The model under review builds one solid part; all positions refer to its coordinate system, in mm. Face numbers are marked on the shaded views. A direction names the side the tool comes from. Round coordinates to 2 decimals unless told otherwise and drop trailing zeros. Order: outer loops, then holes, each group sorted by start corner. A loop starts at its lowest first (then second) coordinate and runs counter-clockwise, first axis right, second up. Notation, with made-up numbers: (-38, 55.5) -> (3, 55.5) arc R16 cw to (3, 63.5) -> close; hole circle Ø10 at (72, -5.75). An arc over 180 degrees is marked (long way). Put each result on its own line as item: value. Start each with the question number.
Autodesk Inventor part; units mm, degrees
ref_plane "YZ Plane" through (0, 0, 0) normal (1, 0, 0) x (0, 1, 0)
ref_plane "XZ Plane" through (0, 0, 0) normal (0, 1, 0) x (-1, 0, 0)
ref_plane "XY Plane" through (0, 0, 0) normal (0, 0, 1) x (1, 0, 0)
sketch "Sketch1" plane through (0, 0, 0) normal (0, 0, 1) x (1, 0, 0)
  line L0 (-15.978, -4.8) -> (15.978, -4.8)
  line L1 (15.978, -4.8) -> (15.978, 4.8)
  line L2 (15.978, 4.8) -> (-15.978, 4.8)
  line L3 (-15.978, 4.8) -> (-15.978, -4.8)
  line L4 (-15.978, -4.8) -> (15.978, 4.8) construction
  line L5 (15.978, -4.8) -> (-15.978, 4.8) construction
  point P0 (0, 0)
  dimension "d0" = 31.956
  dimension "d1" = 9.6
extrude "Extrusion1" add sketch "Sketch1" along normal mid plane 15.928
sketch "Sketch2" plane through (-15.978, 4.8, 7.964) normal (0, 1, 0) x (1, 0, 0)
  circle A0 centre (3.957, 3.957) radius 2.45
  point P0 (15.978, 7.964)
  dimension "d4" = 4.9
extrude "Extrusion2" add sketch "Sketch2" along normal blind 2.1
pattern_linear "Rectangular Pattern1" count 4 spacing 8.014 along (1, 0, 0) of "Extrusion2"
mirror "Mirror1" about plane through (0, 0, 0) normal (0, 0, 1) of "Extrusion2", "Rectangular Pattern1"
sketch "Sketch3" plane through (-12.021, 6.9, 4.007) normal (0, 1, 0) x (1, 0, 0)
  point P0 (12.021, 4.007)
shell "Shell1" thickness 1.557 removed faces 1 at (-5.326, -4.8, 2.6547)
sketch "Sketch4" plane through (-15.978, -4.8, 7.964) normal (0, -1, 0) x (1, 0, 0)
  point P0 (15.978, -7.964)
sketch "Sketch6" plane through (-14.421, 3.243, -6.407) normal (0, -1, 0) x (1, 0, 0)
  circle A0 centre (22.435, 6.407) radius 3.267
  circle A1 centre (22.435, 6.407) radius 2.467
  point P0 (14.421, 6.407)
  point P1 (30.399, -1.557)
  dimension "d13" = 6.534
  dimension "d14" = 0.8
extrude "Extrusion3" add sketch "Sketch6" along normal blind 3
pattern_linear "Rectangular Pattern2" count 3 spacing 8.014 along (-1, 0, 0) of "Extrusion3"
properties part number "Lego Brick"
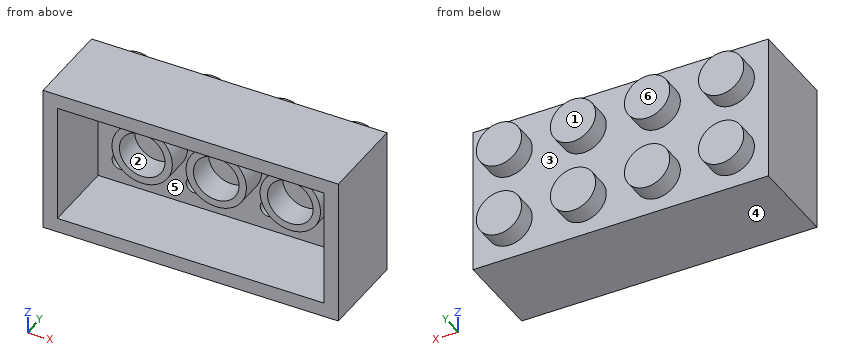
Q1. Draft analysis for pull direction Z (two halves, no side actions). For the marked faces 4, 5 and 6, state which applies: +Z half, -Z half, draft (parallel to the pull), parting line (faces both ways), or undercut.
Q2. For the marked faces 1, 2 and 3, list the 3-axis set-ups (+Z, -Z, +X, -X, +Y, -Y) from which the entire face can be reached by the end or side of a thin tool; tool diameter is ignored.
Q3. Take a section at A-A on y = 1.5. Give the boundary of the cut face in (x, z).
Q4. Wall thickness on probe 1 along Z at (x, y) = (0, 1.9); probe 2 along X at (y, z) = (-1.25, -2.25); probe 3 along Z at (x, y) = (11.5, -3): over which ranges is each line inside the solid? List them lowest first. Write a range as [from, to].
Q5. Take a section at C-C on y = -2.5. Give the boundary of the cut face in (x, z), and give its area (3 significant figures).
Q6. Clearance check with flat-ended pins moving along their axes: pin 1 Ø1.5 at (x, z) = (-8.5, -1) entering from -Y; pin 2 Ø4.5 at (x, z) = (0, 0) entering from +Y; pin 3 Ø1.4 at (x, z) = (4, -4) entering from -Y. State where each tip first meets the part, or that it passes through.
Q7. Take a section at B-B on x = 0. Give the boundary of the cut face in (y, z).
Calculated:
1. face 4: -Z half
1. face 5: undercut
1. face 6: draft
2. face 1: +Z, -Z, +X, -X, +Y
2. face 2: -Y
2. face 3: +Y
3. outline: (-15.98, -7.96) -> (15.98, -7.96) -> (15.98, 7.96) -> (-15.98, 7.96) -> close; circle Ø6.53 at (-8.01, 0); circle Ø6.53 at (0, 0); circle Ø6.53 at (8.01, 0); hole (-14.42, -6.41) -> (14.42, -6.41) -> (14.42, 6.41) -> (-14.42, 6.41) -> close; hole circle Ø4.93 at (-8.01, 0); hole circle Ø4.93 at (0, 0); hole circle Ø4.93 at (8.01, 0)
4. probe 1: z = [-7.96, -6.41], [-3.27, -2.47], [2.47, 3.27], [6.41, 7.96]
4. probe 2: x = [-15.98, -14.42], [14.42, 15.98]
4. probe 3: z = [-7.96, -6.41], [6.41, 7.96]
5. outline: (-15.98, -7.96) -> (15.98, -7.96) -> (15.98, 7.96) -> (-15.98, 7.96) -> close; hole (-14.42, -6.41) -> (14.42, -6.41) -> (14.42, 6.41) -> (-14.42, 6.41) -> close
5. area: 139 mm²
6. pin 1: stops at y = 3.24
6. pin 2: stops at y = 4.8
6. pin 3: stops at y = 5.34
7. outline: (-4.8, -7.96) -> (4.8, -7.96) -> (4.8, 7.96) -> (-4.8, 7.96) -> (-4.8, 6.41) -> (3.24, 6.41) -> (3.24, 3.27) -> (0.24, 3.27) -> (0.24, 2.47) -> (3.24, 2.47) -> (3.24, -2.47) -> (0.24, -2.47) -> (0.24, -3.27) -> (3.24, -3.27) -> (3.24, -6.41) -> (-4.8, -6.41) -> close
